from build123d import *

# Parameters (mm, degrees)
BASE_FLANGE1_DEPTH = 69.85
EDGE_FLANGE1_DEPTH = 275.783864678
EDGE_FLANGE2_DEPTH = 275.783864678
CUT_EXTRUDE1_REACH = 440.752
SKETCH12_W         = 9.573642834
SKETCH12_H         = 76.2


# Sheet-metal steps are written as plain solids
with BuildPart() as part:
    # Sketch1 → Base-Flange1 (new body)
    with BuildSketch(Plane(origin=(0, 0, 0), x_dir=(0, 0, -1), z_dir=(1, 0, 0))):
        with BuildLine():
            Line((0, 0), (0, 275.783864678))
            ThreePointArc((0, 275.783864678), (0.104406833, 276.308753274), (0.401732339, 276.753732339))
            Line((0.401732339, 276.753732339), (134.703841816, 411.055841816))
            Line((134.703841816, 411.055841816), (135.152854622, 410.60682901))
            Line((135.152854622, 410.60682901), (0.850745145, 276.304719533))
            ThreePointArc((0.850745145, 276.304719533), (0.691070336, 276.065749294), (0.635, 275.783864678))
            Line((0.635, 275.783864678), (0.635, 0))
            Line((0.635, 0), (0, 0))
        make_face()
    extrude(amount=BASE_FLANGE1_DEPTH)

    # Edge-Flange1 section (across the edge) → Edge-Flange1 (add)
    with BuildSketch(Plane(origin=(-0.7366, 275.783864678, 0), x_dir=(1, 0, 0), z_dir=(0, -1, 0))):
        with BuildLine():
            Line((-0.635, 0.7366), (-0.635, 62.865))
            Line((-0.635, 62.865), (0, 62.865))
            Line((0, 62.865), (0, 0.7366))
            ThreePointArc((0, 0.7366), (0.215745145, 0.215745145), (0.7366, 0))
            Line((0.7366, 0), (0.7366, -0.635))
            ThreePointArc((0.7366, -0.635), (-0.233267661, -0.233267661), (-0.635, 0.7366))
        make_face()
    extrude(amount=EDGE_FLANGE1_DEPTH)

    # Edge-Flange2 section (across the edge) → Edge-Flange2 (add)
    with BuildSketch(Plane(origin=(70.5866, 0, 0), x_dir=(-1, 0, 0), z_dir=(0, 1, 0))):
        with BuildLine():
            Line((-0.635, 0.7366), (-0.635, 24.765))
            Line((-0.635, 24.765), (0, 24.765))
            Line((0, 24.765), (0, 0.7366))
            ThreePointArc((0, 0.7366), (0.215745145, 0.215745145), (0.7366, 0))
            Line((0.7366, 0), (0.7366, -0.635))
            ThreePointArc((0.7366, -0.635), (-0.233267661, -0.233267661), (-0.635, 0.7366))
        make_face()
    extrude(amount=EDGE_FLANGE2_DEPTH)

    # Sketch12 → Cut-Extrude1 (cut, up to next)
    with BuildSketch(Plane.ZY.offset(1.3716), mode=Mode.PRIVATE) as cut_extrude1_sk1:
        with Locations((58.078178583, 92.075)):
            Rectangle(SKETCH12_W, SKETCH12_H)
    cut_extrude1_tool1 = extrude(cut_extrude1_sk1.sketch, amount=-CUT_EXTRUDE1_REACH, mode=Mode.PRIVATE) & part.part
    add(cut_extrude1_tool1.solids().sort_by_distance((-1.3716, 92.075, 58.078179))[0], mode=Mode.SUBTRACT)


solid = part.part
Could you check a few things on this model? Use its own coordinates, in mm. A direction names the side the tool comes from. Give positions to 0.01 mm unless a question says otherwise; leave off trailing zeros. Order: outer loops, then holes, each group sorted by start corner. A loop starts at its lowest first (then second) coordinate and runs counter-clockwise, first axis right, second up. Notation, with made-up numbers: (83, 68.5) - (109, 68.5) arc R19 ccw to (109, 91.5) - close; hole circle Ø10 at (46, 1.25). An arc over 180 degrees is marked (long way). Return JSON: item names as keys, results as strings. Group by question number.
Q1. Thinking about a two-plate mould opening in X: for faces 1 (the face through (-1.372, 140, 31)), 2 (the face through (34.436, 344.396, -68.942)), 3 (the face through (69.85, 344, -68)), 4 (the face through (-0.737, 140, 32)), which applies, pulls with the +X half, pulls with the -X half, needs draft (parallel to the pull), parting line crosses it, or undercut?
Q2. Will these pins go through, and if not, where does the flat tip stop? pin 1 Ø2 at (x, z) = (30, -53.5) entering from -Y; pin 2 Ø1 at (x, y) = (60.5, 265) entering from +Z; pin 3 Ø1 at (x, y) = (60, 361.5) entering from +Z.
Q3. Suppose I cut it at C-C, the plane y = 214.5. Please give me the cut outline in (x, z) (3 decimals), and give its area (3 significant figures).
Q4. Suppose I cut it at D-D, the plane z = -15. Please give me the cut outline in (x, y), and give its area (3 significant figures).
Q5. Which directions (+Z, -Z, +X, -X, +Y, -Y) give clear straight access to the entire face, cutting with the end or side of a thin tool? Please do faces 5 (the face through (34, 140, -0.635)), 6 (the face through (70.587, 136, 13)), 7 (the face through (34.44, 342.96, -66.61)).
Q6. Suppose I cut it at B-B, the plane x = 59. Please give me the cut outline in (y, z) (3 decimals).
Q7. Suppose I cut it at A-A, the plane z = 15. Please give me the cut outline in (x, y), and give its area (3 significant figures).
Q8. Please list where these lines run through material, in increasing order: line 1 along Z through (x, y) = (25, 30) (3 decimals); line 2 along X through (y, z) = (87.5, 47); line 3 along Z through (x, y) = (12.5, 357.5). Write a range as [from, to].
Resolved:
{
 "1": {"face 1": "pulls with the -X half", "face 2": "needs draft", "face 3": "pulls with the +X half", "face 4": "undercut"},
 "2": {"pin 1": "stops at y = 327.95", "pin 2": "stops at z = 0", "pin 3": "stops at z = -84.65"},
 "3": {"outline": "(-1.372, 0.737) arc R1.372 ccw to (0, -0.635) - (69.85, -0.635) arc R1.372 ccw to (71.222, 0.737) - (71.222, 24.765) - (70.587, 24.765) - (70.587, 0.737) arc R0.737 cw to (69.85, 0) - (0, 0) arc R0.737 cw to (-0.737, 0.737) - (-0.737, 62.865) - (-1.372, 62.865) - close", "area": "101 mm2"},
 "4": {"outline": "(0, 290.45) - (69.85, 290.45) - (69.85, 291.35) - (0, 291.35) - close", "area": "62.7 mm2"},
 "5": {"face 5": "-Z, +X, -X, -Y", "face 6": "+Z, +Y, -Y", "face 7": "+Z, +X, -X, +Y"},
 "6": {"outline": "(0, -0.635) - (275.784, -0.635) arc R0.737 cw to (276.305, -0.851) - (410.607, -135.153) - (411.056, -134.704) - (276.754, -0.402) arc R1.372 ccw to (275.784, 0) - (0, 0) - close"},
 "7": {"outline": "(-1.37, 0) - (-0.74, 0) - (-0.74, 275.78) - (-1.37, 275.78) - close; (70.59, 0) - (71.22, 0) - (71.22, 275.78) - (70.59, 275.78) - close", "area": "350 mm2"},
 "8": {"line 1": "z = [-0.635, 0]", "line 2": "x = [-1.37, -0.74]", "line 3": "z = [-82.05, -81.15]"}
}
